Can you work these out from the model? Positions are in its coordinate system, mm. A direction names the side the tool comes from. Give positions to 0.01 mm unless a question says otherwise; leave off trailing zeros. Write each loop counter-clockwise with the first axis right and the second up, starting at its lowest first coordinate (ties: lowest second). Pieces come first, ordered by that corner, then holes. Notation, with made-up numbers: (18.25, -30) -> (54.25, -30) arc R10 ccw to (54.25, -14) -> close; hole circle Ø8 at (89.25, 57.25). An arc over 180 degrees is marked (long way). One line per item, written item: value.
from build123d import *

# Parameters (mm, degrees)
BOSS_EXTRUDE1_DEPTH      = 14
BOSS_EXTRUDE2_DEPTH      = 12
BOSS_EXTRUDE2_DEPTH_BACK = 12
CUT_EXTRUDE1_DEPTH       = 20
FILLET1_R                = 4
SKETCH5_R                = 10
BOSS_EXTRUDE3_DEPTH      = 24
SKETCH6_R                = 10
CUT_EXTRUDE2_DEPTH       = 78


with BuildPart() as part:
    # Sketch1 → Boss-Extrude1 (new body)
    with BuildSketch(Plane(origin=(0, 0, 0), x_dir=(1, 0, 0), z_dir=(0, 1, 0))):
        with BuildLine():
            Line((-24, 12), (-24, -12))
            Line((-24, -12), (-23.832750576, -12))
            ThreePointArc((-23.832750576, -12), (-17.627403759, -13.013689636), (-12.067215481, -15.949367089))
            ThreePointArc((-12.067215481, -15.949367089), (20, 0), (-12.067215481, 15.949367089))
            ThreePointArc((-12.067215481, 15.949367089), (-17.627403759, 13.013689636), (-23.832750576, 12))
            Line((-23.832750576, 12), (-24, 12))
        make_face()
    boss_extrude1 = extrude(amount=BOSS_EXTRUDE1_DEPTH)

    # Sketch3 → Boss-Extrude2 (add, two sides: drawn at the far end of the back side and taken through both)
    with BuildSketch(Plane.XY.offset(-BOSS_EXTRUDE2_DEPTH_BACK)):
        with BuildLine():
            Line((-46.897875765, 0), (-119.832750576, 0))
            Line((-119.832750576, 0), (-119.832750576, -24))
            Line((-119.832750576, -24), (-46.897875765, -24))
            ThreePointArc((-46.897875765, -24), (-37.323488139, -34.226110771), (-23.832750576, -38))
            Line((-23.832750576, -38), (-23.832750576, -24))
            ThreePointArc((-23.832750576, -24), (-35.832750576, -12), (-23.832750576, 0))
            Line((-23.832750576, 0), (-23.832750576, 14))
            ThreePointArc((-23.832750576, 14), (-37.323488139, 10.226110771), (-46.897875765, 0))
        make_face()
    extrude(amount=BOSS_EXTRUDE2_DEPTH + BOSS_EXTRUDE2_DEPTH_BACK)

    # Sketch4 → Cut-Extrude1 (cut)
    with BuildSketch(Plane.ZY.offset(119.832750576)):
        Polygon((-12, 0), (-4, 0), (-12, -8), align=None)
        Polygon((4, 0), (12, -8), (12, 0), align=None)
        Polygon((12, -16), (4, -24), (12, -24), align=None)
        Polygon((-4, -24), (-12, -16), (-12, -24), align=None)
    extrude(amount=-CUT_EXTRUDE1_DEPTH, mode=Mode.SUBTRACT)

    # Fillet1
    fillet1_edges = [part.edges().sort_by_distance(p)[0] for p in [
        (-99.832750576, -20, -8),
        (-99.832750576, -20, 8),
        (-99.832750576, -4, 8),
        (-99.832750576, -4, -8),
    ]]
    fillet(fillet1_edges, radius=FILLET1_R)

    # Sketch5 → Boss-Extrude3 (add)
    with BuildSketch(Plane.ZY.offset(119.832750576)):
        with Locations((0, -12)):
            Circle(SKETCH5_R)
    extrude(amount=BOSS_EXTRUDE3_DEPTH)

    # Mirror1: Boss-Extrude1 across plane
    add(boss_extrude1.mirror(Plane.ZX.offset(-12)))

    # Sketch6 → Cut-Extrude2 (cut)
    with BuildSketch(Plane(origin=(0, 14, 0), x_dir=(1, 0, 0), z_dir=(0, 1, 0))):
        with Locations(Location((0, 0, 0), (0, 0, 90))):
            Circle(SKETCH6_R)
    extrude(amount=-CUT_EXTRUDE2_DEPTH, mode=Mode.SUBTRACT)


solid = part.part
1) We'd pull the mould along Z, two halves only. Please class faces 1 (the face through (-112, -4, -8)), 2 (the face through (9.76, -30.9, 2.17)), 3 (the face through (-132, -18, -8)): released by +Z, released by -Z, zero draft, split by the parting line, or undercut.
Answer list:
face 1: released by -Z
face 2: undercut
face 3: split by the parting line
2) If we section it at C-C (y = 8): Write out the boundary of the cut face in (x, z), and give its area (3 significant figures).
Answer list:
outline: (-40.45, -12) -> (-23.83, -12) arc R19.5 cw to (-12.07, -15.95) arc R20 ccw (long way) to (-12.07, 15.95) arc R19.5 cw to (-23.83, 12) -> (-40.45, 12) -> close; hole circle Ø20 at (0, 0)
area: 1,480 mm^2
3) If we section it at A-A (x = 0): Write out the boundary of the cut face in (y, z), and give its area (3 significant figures).
Answer list:
outline: (-38, -20) -> (-24, -20) -> (-24, -10) -> (-38, -10) -> close; (-38, 10) -> (-24, 10) -> (-24, 20) -> (-38, 20) -> close; (0, -20) -> (14, -20) -> (14, -10) -> (0, -10) -> close; (0, 10) -> (14, 10) -> (14, 20) -> (0, 20) -> close
area: 560 mm^2
4) If we section it at D-D (x = -114.5): Write out the boundary of the cut face in (y, z).
Answer list:
outline: (-24, -4) -> (-16, -12) -> (-8, -12) -> (0, -4) -> (0, 4) -> (-8, 12) -> (-16, 12) -> (-24, 4) -> close
5) If we section it at B-B (z = 0): State how many separate pieces and enclosed holes the cut face has, and give its area (3 significant figures).
Answer list:
separate pieces: 3
enclosed holes: 0
area: 3,690 mm^2
6) I need wall thicknesses on L1, parallel to Y at x = -68.5, z = 9; L2, parallel to Y at x = -13, z = 4; L3, parallel to Z at x = -29.5, y = -26.5. Which ranges of each line are inside material? Lowest first, please.
Answer list:
L1: y = -24 to 0
L2: y = -38 to -24, 0 to 14
L3: z = -12 to 12
7) For faces 4 (the face through (-62, -12, -12)), 5 (the face through (-76, -24, 0)), 6 (the face through (-12, 0, 0)), which set-ups out of +Z, -Z, +X, -X, +Y, -Y let a thin tool reach every point of the face, with its end or its side?
Answer list:
face 4: -Z, -X, +Y, -Y
face 5: +Z, -Z, -X, -Y
face 6: +Z, -Z, +X
8) Will these pins go through, and if not, where does the flat tip stop? pin 1 (5 mm diameter, centred on x = -30.5, y = -29, fed in from -Z); pin 2 (18 mm diameter, centred on x = 0, z = 0, fed in from +Y); pin 3 (5 mm diameter, centred on x = -127.5, z = 1, fed in from +Y); pin 4 (1.2 mm diameter, centred on y = -23.5, z = -11, fed in from -X).
Answer list:
pin 1: stops at z = -12
pin 2: passes through
pin 3: stops at y = -2
pin 4: stops at x = -99.83
